Part model, mm, in its own coordinate system. A direction names the side the tool comes from. Give positions to 0.01 mm unless a question says otherwise; leave off trailing zeros. Order: outer loops, then holes, each group sorted by start corner. A loop starts at its lowest first (then second) coordinate and runs counter-clockwise, first axis right, second up.
from build123d import *

# Parameters (mm, degrees)
F1_DEPTH = 10
F2_R     = 1.6
F3_DEPTH = 4.601
F4_DEPTH = 3
F5_R     = 0.5


with BuildPart() as f1:
    # F0 (on Top) → F1 (new body)
    with BuildSketch(Plane.XY):
        Polygon((-2.9, 2), (-5, 2), (-2.5, -2), (2.5, -2), (5, 2), (2.9, 2), (2.9, 2.6), (-2.9, 2.6), align=None)
    extrude(amount=F1_DEPTH)

    # F2 (on face) → F3 (cut, through all)
    with BuildSketch(Plane.XZ.offset(2)):
        with Locations((0, 5)):
            Circle(F2_R)
    extrude(amount=-F3_DEPTH, mode=Mode.SUBTRACT)

    # F2 (on face) → F4 (cut)
    with BuildSketch(Plane.XZ.offset(2)):
        Polygon((0, 1.651368), (2.5, 3.094744), (2.5, 6.905256), (0, 8.348632), (-2.5, 6.905256), (-2.5, 3.094744), align=None)
        with Locations((0, 5)):
            Circle(F2_R, mode=Mode.SUBTRACT)
        Polygon((2.5, 3.094744), (2.9, 3.325684), (2.9, 6.674316), (2.5, 6.905256), align=None)
        Polygon((-2.9, 3.325684), (-2.5, 3.094744), (-2.5, 6.905256), (-2.9, 6.674316), align=None)
    extrude(amount=-F4_DEPTH, mode=Mode.SUBTRACT)

    # F5
    f5_edges = [f1.edges().sort_by_distance(p)[0] for p in [
        (-5, 2, 5),
        (-2.5, -2, 1.547372),
        (-2.5, -2, 8.452628),
        (2.5, -2, 1.547372),
        (2.5, -2, 8.452628),
        (5, 2, 5),
        (-2.9, 2.6, 5),
        (2.9, 2.6, 5),
    ]]
    fillet(f5_edges, radius=F5_R)


solid = f1.part
Item 1: Band-saw the part on C-C on x = 1.25. List the corners of the cut face in (y, z), plus the area to 3 significant figures.
Item 2: Drill centre lines: probe 1 along Z at (x, y) = (0, 1.55); probe 2 along Z at (x, y) = (2.5, -0.2); probe 3 along X at (y, z) = (-1.2, 2.75). Where is each one in solid material? Low to high.
Item 3: Band-saw the part on B-B on z = 5. List the corners of the cut face in (x, y) (3 decimals).
Item 4: Which spindle directions (+Z, -Z, +X, -X, +Y, -Y) get a long thin tool onto all of the face, cutting with end or side? Do faces 4 (the face through (1, 1, 7)), 5 (the face through (-3.5, 2, 4.9)), 6 (the face through (-3.6, -0.24, 4.93)). Say none if no direction does.
Item 5: Band-saw the part on A-A on y = 0.8. List the corners of the cut face in (x, z), plus the area to 3 significant figures.
Item 6: Band-saw the part on D-D on y = 0. List the corners of the cut face in (x, z), plus the area to 3 significant figures.
Item 7: Drop flat-ended pins along their axis: P1, Ø5, axis at x = 0, z = 5, coming from the -Y side; P2, Ø1, axis at x = 3.5, z = 3.5, coming from the +Y side; P3, Ø1.2, axis at y = 0, z = 4.5, coming from the -X side (3 decimals). Give the stop position or say it passes through.
Item 8: Pull direction X, two halves, no side cores. Call faces 1 (the face through (3.57, -0.29, 4.93)), 2 (the face through (2.9, 0, 5)), 3 (the face through (3.5, 2, 4.9)): released by +X, released by -X, zero draft, split by the parting line, or undercut.
Working result:
1. outline: (-2, 0) - (2.6, 0) - (2.6, 4) - (1, 4) - (1, 2.37) - (-2, 2.37) - close; (-2, 7.63) - (1, 7.63) - (1, 6) - (2.6, 6) - (2.6, 10) - (-2, 10) - close
1. area: 27.0 mm2
2. probe 1: z = 0 to 3.4, 6.6 to 10
2. probe 2: z = 0 to 3.09, 6.91 to 10
2. probe 3: x = -3 to -1.9, 1.9 to 3
3. outline: (-4.522, 1.235) - (-2.9, -1.36) - (-2.9, 1) - (-1.6, 1) - (-1.6, 2.6) - (-2.4, 2.6) arc R0.5 ccw to (-2.9, 2.1) - (-2.9, 2) - (-4.098, 2) arc R0.5 ccw to start; (1.6, 1) - (2.9, 1) - (2.9, -1.36) - (4.522, 1.235) arc R0.5 ccw to (4.098, 2) - (2.9, 2) - (2.9, 2.1) arc R0.5 ccw to (2.4, 2.6) - (1.6, 2.6) - close
4. face 4: -Y
4. face 5: +Z, -Z, -X, +Y
4. face 6: +Z, -Z, -X, -Y
5. outline: (-4.25, 0) - (4.25, 0) - (4.25, 10) - (-4.25, 10) - close; hole (-2.9, 3.33) - (-2.5, 3.09) - (0, 1.65) - (2.5, 3.09) - (2.9, 3.33) - (2.9, 6.67) - (2.5, 6.91) - (0, 8.35) - (-2.5, 6.91) - (-2.9, 6.67) - close
5. area: 55.9 mm2
6. outline: (-3.75, 0) - (3.75, 0) - (3.75, 10) - (-3.75, 10) - close; hole (-2.9, 3.33) - (-2.5, 3.09) - (0, 1.65) - (2.5, 3.09) - (2.9, 3.33) - (2.9, 6.67) - (2.5, 6.91) - (0, 8.35) - (-2.5, 6.91) - (-2.9, 6.67) - close
6. area: 45.9 mm2
7. P1: stops at y = 1
7. P2: stops at y = 2
7. P3: stops at x = -4.125
8. face 1: released by +X
8. face 2: undercut
8. face 3: zero draft
